from build123d import *

# Parameters (mm, degrees)
SKETCH_1_W          = 11.5
SKETCH_1_H          = 23
EXTRUDE_1_DEPTH     = 19.65
SKETCH_3_W          = 11.5
SKETCH_3_H          = 32
EXTRUDE_3_DEPTH     = 1.36
SKETCH_4_R          = 1
CUT_EXTRUDE_1_DEPTH = 5
FILLET_8_R          = 2
SKETCH_9_R          = 5.75
EXTRUDE_7_DEPTH     = 4
SKETCH_10_R         = 2
EXTRUDE_8_DEPTH     = 3


with BuildPart() as part:
    # 草图1 → 凸台-拉伸1 (new body)
    with BuildSketch(Plane(origin=(0, 0, 0), x_dir=(1, 0, 0), z_dir=(0, 1, 0))):
        Rectangle(SKETCH_1_W, SKETCH_1_H)
    extrude(amount=EXTRUDE_1_DEPTH)

    # 草图3 → 凸台-拉伸3 (add)
    with BuildSketch(Plane(origin=(0, 15, 0), x_dir=(-1, 0, 0), z_dir=(0, -1, 0))):
        Rectangle(SKETCH_3_W, SKETCH_3_H)
    extrude(amount=-EXTRUDE_3_DEPTH)

    # 草图4 → 切除-拉伸1 (cut)
    with BuildSketch(Plane(origin=(0, 15, 0), x_dir=(-1, 0, 0), z_dir=(0, -1, 0))):
        with Locations(Location((0, 13.8, 0), (0, 0, 90))):
            Circle(SKETCH_4_R)
        with Locations(Location((0, -13.8, 0), (0, 0, 90))):
            Circle(SKETCH_4_R)
    extrude(amount=-CUT_EXTRUDE_1_DEPTH, mode=Mode.SUBTRACT)

    # 圆角8
    fillet_8_edges = [part.edges().sort_by_distance(p)[0] for p in [
        (-5.75, 15.68, -16),
        (5.75, 15.68, 16),
        (-5.75, 15.68, 16),
        (5.75, 15.68, -16),
    ]]
    fillet(fillet_8_edges, radius=FILLET_8_R)

    # 草图9 → 凸台-拉伸7 (add)
    with BuildSketch(Plane(origin=(0, 19.65, 0), x_dir=(1, 0, 0), z_dir=(0, 1, 0))):
        with Locations(Location((0, -5.75, 0), (0, 0, 270))):
            Circle(SKETCH_9_R)
    extrude(amount=EXTRUDE_7_DEPTH)

    # 草图10 → 凸台-拉伸8 (add)
    with BuildSketch(Plane(origin=(0, 23.65, 0), x_dir=(1, 0, 0), z_dir=(0, 1, 0))):
        with Locations(Location((0, -5.75, 0), (0, 0, 270))):
            Circle(SKETCH_10_R)
    extrude(amount=EXTRUDE_8_DEPTH)


solid = part.part
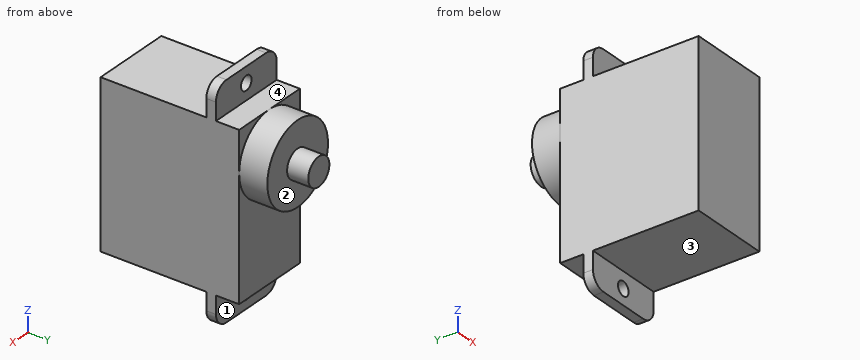
Work out the finished part from the listing and answer in its coordinate system (mm). Face numbers are marked on the shaded views. A direction names the side the tool comes from. Round coordinates to 2 decimals unless told otherwise and drop trailing zeros. Loops run counter-clockwise (first coordinate to the right, second up) from the corner with the lowest first, then second, coordinate; pieces in that order, holes last. Notation, with made-up numbers: M 22,14.25 L 72,14.25 A25 cw 72,38.25 Z; hole C 51,38.5 d1. An arc over 180 degrees is marked long. One line per question, with ' | ' between items. Start each with the question number.
(1) A cutting plane is placed at C-C on y = 17.5. Write down the section's boundary in (x, z), plus the area to 4 significant figures.
(2) Flat-ended cylindrical pins translate along their axes: pin 1 Ø3.5 at (x, y) = (2, 6) entering from -Z; pin 2 Ø1.7 at (x, z) = (4, 7.5) entering from +Y; pin 3 Ø3 at (x, z) = (0, -13.8) entering from -Y; pin 4 Ø1.6 at (x, z) = (0, 13.8) entering from +Y. Find the tip coordinate at first contact, or state that the pin passes through.
(3) A cutting plane is placed at D-D on x = 1.5. Write down the section's boundary in (y, z).
(4) A tool of negligible diameter and unlimited length cuts with its end or side. For the marked faces 1, 2, 3 and 4, from which of +Z, -Z, +X, -X, +Y, -Y can it reach the whole face along a straight path? Write none if from no direction.
(5) A cutting plane is placed at A-A on z = -1. Write down the section's boundary in (x, y).
(6) Find the intervals of material crossed by line 1 (X direction, y = 16.15, z = 13.8); line 2 (Z direction, x = -1, y = 10.5); line 3 (Y direction, x = 2, z = 11), in increasing order.
(7) A cutting plane is placed at B-B on x = -2.5. Write down the section's boundary in (y, z), plus the area to 3 significant figures.
Geometry check:
1) outline: M -5.75,-11.5 L 5.75,-11.5 L 5.75,11.5 L -5.75,11.5 Z | area: 264.5 mm²
2) pin 1: stops at z = -11.5 | pin 2: stops at y = 23.65 | pin 3: stops at y = 15 | pin 4: passes through
3) outline: M 0,-11.5 L 15,-11.5 L 15,-16 L 16.36,-16 L 16.36,-11.5 L 19.65,-11.5 L 19.65,0.2 L 23.65,0.2 L 23.65,4.43 L 26.65,4.43 L 26.65,7.07 L 23.65,7.07 L 23.65,11.3 L 19.65,11.3 L 19.65,11.5 L 16.36,11.5 L 16.36,16 L 15,16 L 15,11.5 L 0,11.5 Z
4) face 1: -Z, +X, -X, +Y | face 2: +Y | face 3: -Z, +X, -X, -Y | face 4: +Z, +X, -X, +Y
5) outline: M -5.75,0 L 5.75,0 L 5.75,19.65 L -5.75,19.65 Z
6) line 1: x = -5.75 to -1, 1 to 5.75 | line 2: z = -11.5 to 11.5 | line 3: y = 0 to 23.65
7) outline: M 0,-11.5 L 15,-11.5 L 15,-16 L 16.36,-16 L 16.36,-11.5 L 19.65,-11.5 L 19.65,0.57 L 23.65,0.57 L 23.65,10.93 L 19.65,10.93 L 19.65,11.5 L 16.36,11.5 L 16.36,16 L 15,16 L 15,11.5 L 0,11.5 Z | area: 506 mm²
